Model file for the job. Use its own axes, mm. Round coordinates to 2 decimals unless told otherwise and drop trailing zeros. Loops run counter-clockwise (first coordinate to the right, second up) from the corner with the lowest first, then second, coordinate; pieces in that order, holes last. Notation, with made-up numbers: (41.5, 47) - (65.5, 47) arc R24 cw to (65.5, 63) - close; hole circle Ø11 at (33, -2.75). An arc over 180 degrees is marked (long way). Use one line per item in the form item = value.
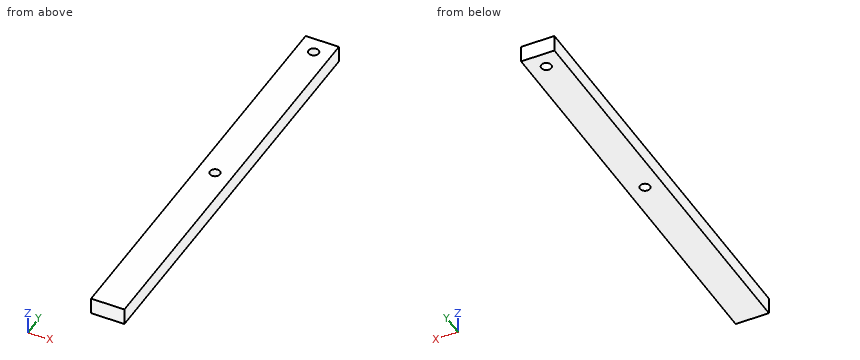
from build123d import *

# Parameters (mm, degrees)
SKETCH1_W           = 20
SKETCH1_H           = 250
BOSS_EXTRUDE1_DEPTH = 10
SKETCH2_R           = 3
CUT_EXTRUDE1_DEPTH  = 10


with BuildPart() as part:
    # Sketch1 → Boss-Extrude1 (new body)
    with BuildSketch(Plane.XY):
        Rectangle(SKETCH1_W, SKETCH1_H)
    extrude(amount=BOSS_EXTRUDE1_DEPTH)

    # Sketch2 → Cut-Extrude1 (cut)
    with BuildSketch(Plane.XY.offset(10)):
        with Locations((0, 115)):
            Circle(SKETCH2_R)
        Circle(SKETCH2_R)
    extrude(amount=-CUT_EXTRUDE1_DEPTH, mode=Mode.SUBTRACT)


solid = part.part
1. Flat gauge pin, fed straight in: pin 1 (6 mm diameter, centred on x = 1, y = -61.5, fed in from -Z). Where does the tip first touch, or does it go through?
Geometry check:
pin_1 = 0
2. Cut at B-B, the plane y = 0. Give the cut face in (x, z), plus the area to 3 significant figures.
Geometry check:
outline = (-10, 0) - (-3, 0) - (-3, 10) - (-10, 10) - close; (3, 0) - (10, 0) - (10, 10) - (3, 10) - close
area = 140 mm^2
3. Cut at A-A, the plane x = 0. Give the cut face in (y, z), plus the area to 3 significant figures.
Geometry check:
outline = (-125, 0) - (-3, 0) - (-3, 10) - (-125, 10) - close; (3, 0) - (112, 0) - (112, 10) - (3, 10) - close; (118, 0) - (125, 0) - (125, 10) - (118, 10) - close
area = 2,380 mm^2
4. Wall check: probe 1 along Y at (x, z) = (0, 3); probe 2 along Y at (x, z) = (-2.5, 9.25). Give the ranges that are in metal, low to high.
Geometry check:
probe_1 = -125 to -3, 3 to 112, 118 to 125
probe_2 = -125 to -1.66, 1.66 to 113.34, 116.66 to 125
